Autodesk Inventor part; units mm, degrees
ref_plane "YZ Plane" through (0, 0, 0) normal (1, 0, 0) x (0, 1, 0)
ref_plane "XZ Plane" through (0, 0, 0) normal (0, 1, 0) x (-1, 0, 0)
ref_plane "XY Plane" through (0, 0, 0) normal (0, 0, 1) x (1, 0, 0)
sketch "Эскиз1" plane through (0, 0, 0) normal (0, 0, 1) x (1, 0, 0)
  line L0 (-12.5, 120) -> (12.5, 120)
  line L1 (12.5, 120) -> (12.5, -130)
  line L2 (12.5, -130) -> (-12.5, -130)
  line L3 (-12.5, -130) -> (-12.5, 120)
  line L4 (-17.5, 0) -> (17.5, 0)
  line L5 (0, -180) -> (0, 170)
  point P0 (0, 0)
  dimension "d0" = 250
  dimension "d1" = 25
  dimension "d2" = 120
extrude "Выдавливание1" add sketch "Эскиз1" along normal blind 100 and the other way blind 120
sketch "Эскиз2" plane through (12.5, -130, 100) normal (1, 0, 0) x (0, 0, -1)
  line L0 (0, 250) -> (220, 250)
  line L1 (0, 0) -> (0, 250)
  line L2 (220, 250) -> (220, 0)
  line L3 (0, 0) -> (220, 0)
  line L4 (6, 244) -> (214, 244)
  line L5 (214, 244) -> (214, 6)
  line L6 (214, 6) -> (6, 6)
  line L7 (6, 6) -> (6, 244)
  point P0 (100, 130)
  dimension "d7" = 6
  dimension "d8" = 6
  dimension "d9" = 6
  dimension "d10" = 6
extrude "Выдавливание2" cut sketch "Эскиз2" against normal through all contours L4 L5 L6 L7
fillet "Сопряжение1" radius 15 4 edges at (0, 120, 100) (0, 120, -120) (0, -130, 100) (0, -130, -120)
sketch "Эскиз3" plane through (12.5, -115, -120) normal (1, 0, 0) x (0, 0, -1)
  arc A0 (-205, 235) -> (-220, 220) centre (-205, 220) ccw
  arc A1 (0, 220) -> (-15, 235) centre (-15, 220) ccw
  arc A2 (-15, -15) -> (0, 0) centre (-15, 0) ccw
  arc A3 (-220, 0) -> (-205, -15) centre (-205, 0) ccw
  arc A4 (-15, -15) -> (0, 0) centre (-15, 0) ccw
  circle A5 centre (-205, 0) radius 15
  circle A6 centre (-15, 0) radius 15
  circle A7 centre (-15, 220) radius 15
  circle A8 centre (-205, 220) radius 15
  point P0 (-120, 115)
  dimension "d15" = 30
extrude "Выдавливание3" add sketch "Эскиз3" against normal up to surface (25 mm away)
fillet "Сопряжение2" radius 5 6 edges at (0, 93, 94) (0, 93, -114) (0, -103, -114) (0, -103, 94) (0, 114, 73) (0, -124, -93)
sketch "Эскиз4" plane through (-12.5, -115, -120) normal (-1, 0, 0) x (0, 0, 1)
  line L0 (0, 0) -> (0, 220)
  arc A0 (0, 0) -> (15, -15) centre (15, 0) ccw
  line L1 (205, -15) -> (15, -15)
  arc A1 (205, -15) -> (220, 0) centre (205, 0) ccw
  line L2 (220, 220) -> (220, 0)
  arc A2 (220, 220) -> (205, 235) centre (205, 220) ccw
  line L3 (15, 235) -> (205, 235)
  arc A3 (15, 235) -> (0, 220) centre (15, 220) ccw
  line L4 (27, 229) -> (185.4041, 229)
  arc A4 (190.3031, 223) -> (208, 205.3031) centre (205, 220) ccw
  arc A5 (214, 200.4041) -> (208, 205.3031) centre (209, 200.4041) ccw
  line L5 (214, 200.4041) -> (214, 19.5959)
  arc A6 (208, 14.6969) -> (214, 19.5959) centre (209, 19.5959) ccw
  arc A7 (208, 14.6969) -> (193, -9) centre (205, 0) ccw
  line L6 (193, -9) -> (34.5959, -9)
  arc A8 (29.6969, -3) -> (12, 14.6969) centre (15, 0) ccw
  arc A9 (6, 19.5959) -> (12, 14.6969) centre (11, 19.5959) ccw
  line L7 (6, 19.5959) -> (6, 200.4041)
  arc A10 (12, 205.3031) -> (6, 200.4041) centre (11, 200.4041) ccw
  arc A11 (12, 205.3031) -> (27, 229) centre (15, 220) ccw
  circle A12 centre (15, 0) radius 5.1
  circle A13 centre (15, 220) radius 5.1
  arc A14 (220, 220) -> (205, 235) centre (205, 220) ccw
  circle A15 centre (205, 220) radius 5.1
  circle A16 centre (205, 0) radius 5.1
  arc A17 (190.3031, 223) -> (185.4041, 229) centre (185.4041, 224) ccw
  arc A18 (29.6969, -3) -> (34.5959, -9) centre (34.5959, -4) ccw
  point P0 (120, 115)
  dimension "d19" = 10.2
extrude "Выдавливание4" cut sketch "Эскиз4" against normal through all contours A12 | A13 | A15 | A16
fillet "Сопряжение4" radius 15 2 edges at (0, 114, -93) (0, -124, 73)
sketch "Эскиз6" plane through (-12.5, -115, -120) normal (-1, 0, 0) x (0, 0, 1)
  circle A0 centre (15, 220) radius 5.1
  circle A1 centre (205, 0) radius 5.1
  circle A2 centre (195, -5) radius 3
  circle A3 centre (25, 225) radius 3
  point P0 (120, 115)
  dimension "d35" = 6
  dimension "d37" = 10
  dimension "d38" = 5
  dimension "d39" = 230
  dimension "d40" = 170
extrude "Выдавливание6" cut sketch "Эскиз6" against normal through all contours A2 | A3
chamfer "Фаска2" distance 0.6 angle 45 4 edges at (-12.5, 110, -98) (-12.5, -120, 72) (12.5, -120, 72) (12.5, 110, -98)
sketch "Эскиз7" plane through (12.5, -115, 100) normal (1, 0, 0) x (0, 0, -1)
  line L0 (15, -15) -> (205, -15)
  line L1 (220, 220) -> (220, 0)
  line L2 (15, 235) -> (205, 235)
  line L3 (220, -15) -> (240, -15)
  line L4 (240, -15) -> (240, 235)
  line L5 (240, 235) -> (220, 235)
  line L6 (220, 235) -> (220, -15)
  line L7 (230, -15) -> (230, 235) construction
  circle A0 centre (230, 5) radius 4.25
  circle A1 centre (230, 75) radius 4.25
  circle A2 centre (230, 145) radius 4.25
  circle A3 centre (230, 215) radius 4.25
  point P0 (100, 115)
  dimension "d46" = 20
  dimension "d49" = 8.5
  dimension "d50" = 20
  dimension "d51" = 70
  dimension "d52" = 20
  dimension "d53" = 70
extrude "Выдавливание7" add sketch "Эскиз7" against normal up to surface (25 mm away) contours L6 L5 L4 L3 L1 | A0 | A1 | A2 | A3
extrude "Выдавливание8" cut sketch "Эскиз7" against normal through all contours A0 | A1 | A2 | A3
properties part number "Корпус03"
The model under review builds one solid part; all positions refer to its coordinate system, in mm. A direction names the side the tool comes from. Coordinates: 2 decimals unless noted, no trailing zeros. Write each loop counter-clockwise with the first axis right and the second up, starting at its lowest first coordinate (ties: lowest second). Pieces come first, ordered by that corner, then holes. Notation, with made-up numbers: (49.25, 11) -> (91.25, 11) arc R16 ccw to (91.25, 23) -> close; hole circle Ø5 at (-25, -6.5). An arc over 180 degrees is marked (long way). One line per item, written item: value. Start each with the question number.
Q1. For faces 4 (the face through (12.5, -4, -117)), 5 (the face through (0.18, -99.24, 92.21)), list the 3-axis set-ups (+Z, -Z, +X, -X, +Y, -Y) from which the entire face can be reached by the end or side of a thin tool; tool diameter is ignored.
Q2. Add section B-B, the plane z = 6. Give the boundary of the cut face in (x, y).
Q3. The part is to be moulded in two halves that separate along Z. For faces 1 (the face through (-12.5, -4, -117)), 2 (the face through (0, 110, -98)), 3 (the face through (0.18, 115.72, 95.49)), say which applies: +Z half, -Z half, draft (parallel to the pull), parting line (faces both ways), or undercut.
Q4. Add section C-C, the plane z = -95. Give the boundary of the cut face in (x, y), then the cut area to 3 significant figures.
Q5. Clearance check with flat-ended pins moving along their axes: P1, Ø5, axis at y = 30, z = -130, coming from the -X side; P2, Ø4.5, axis at x = 4, y = 116, coming from the +Z side; P3, Ø7, axis at y = 110, z = -95, coming from the +X side; P4, Ø7, axis at y = -120, z = 75, coming from the -X side. State where each tip first meets the part, or that it passes through.
Q6. Add section D-D, the plane x = -2.25. Count the separate pieces of the cut face and the enclosed holes in it, then the cut area to 3 significant figures.
Q7. Add section A-A, the plane y = -27. Give the boundary of the cut face in (x, z), then the cut area to 3 significant figures.
Q8. To check wall thickness, follow probe 1 along Y at (x, z) = (4.25, -130); probe 2 along Y at (x, z) = (-1, -105); probe 3 along Y at (x, z) = (-3.5, 52). State the ranges of each line that lie inside material, in increasing order.
Response:
1. face 4: +Z, -Z, +X, +Y, -Y
1. face 5: +X, -X
2. outline: (-12.5, -130) -> (12.5, -130) -> (12.5, -124) -> (-12.5, -124) -> close; (-12.5, 114) -> (12.5, 114) -> (12.5, 120) -> (-12.5, 120) -> close
3. face 1: draft
3. face 2: undercut
3. face 3: +Z half
4. outline: (-12.5, -130) -> (12.5, -130) -> (12.5, -103.82) -> (-12.5, -103.82) -> close; (-12.5, 93.82) -> (12.5, 93.82) -> (12.5, 106.4) -> (11.9, 107) -> (-11.9, 107) -> (-12.5, 106.4) -> close; (-12.5, 113.6) -> (-11.9, 113) -> (11.9, 113) -> (12.5, 113.6) -> (12.5, 120) -> (-12.5, 120) -> close
4. area: 1,160 mm²
5. P1: through
5. P2: z = 97.18
5. P3: x = 12.4
5. P4: x = -12.4
6. separate pieces: 1
6. enclosed holes: 11
6. area: 11,900 mm²
7. outline: (-12.5, -140) -> (12.5, -140) -> (12.5, -114) -> (-12.5, -114) -> close; (-12.5, 94) -> (12.5, 94) -> (12.5, 100) -> (-12.5, 100) -> close
7. area: 800 mm²
8. probe 1: -130 to -114.25, -105.75 to -44.25, -35.75 to 25.75, 34.25 to 95.75, 104.25 to 120
8. probe 2: -130 to -120.1, -109.9 to -100, 90 to 99.9, 110.1 to 120
8. probe 3: -130 to -124, 114 to 120
